Autodesk Inventor part; units mm, degrees
ref_plane "YZ Plane" through (0, 0, 0) normal (1, 0, 0) x (0, 1, 0)
ref_plane "XZ Plane" through (0, 0, 0) normal (0, 1, 0) x (-1, 0, 0)
ref_plane "XY Plane" through (0, 0, 0) normal (0, 0, 1) x (1, 0, 0)
sketch "Szkic2" plane through (0, 0, 0) normal (0, 1, 0) x (-1, 0, 0)
  circle A0 centre (0, 0) radius 11
  circle A1 centre (0, 0) radius 16
  dimension "d0" = 22
  dimension "d1" = 5
extrude "Wyciągnięcie proste1" add sketch "Szkic2" along normal blind 10
sketch "Szkic4" plane through (0, 0, 0) normal (0, 0, 1) x (1, 0, 0)
  line L0 (0, 0) -> (-30, 0)
  line L1 (-30, 0) -> (-30, 10)
  line L2 (-30, 10) -> (0, 10)
  line L3 (0, 10) -> (0, 0)
  line L4 (-30, 0) -> (-40, 0)
  line L5 (-40, 0) -> (-40, 84.8)
  line L6 (-40, 84.8) -> (-30, 84.8)
  line L7 (-30, 84.8) -> (-30, 0)
  dimension "d7" = 84.8
  dimension "d8" = 30
  dimension "d9" = 10
  dimension "d10" = 10
extrude "Wyciągnięcie proste2" add sketch "Szkic4" along normal mid plane 10
fillet "Zaokrąglenie1" radius 20 2 edges at (-40, 0, 0) (-30, 10, 0)
sketch "Szkic7" plane through (-30, 84.8, 5) normal (1, 0, 0) x (0, 0, -1)
  line L0 (10, 0) -> (0, 0)
  circle A0 centre (5, 0) radius 11
  circle A1 centre (5, 0) radius 16
  point P0 (5, -84.8)
  dimension "d14" = 22
  dimension "d15" = 32
extrude "Wyciągnięcie proste3" add sketch "Szkic7" against normal blind 10
sketch "Szkic8" plane through (0, 10, 0) normal (0, 1, 0) x (1, 0, 0)
  circle A0 centre (0, 0) radius 11
extrude "Wyciągnięcie proste4" cut sketch "Szkic8" against normal blind 10
sketch "Szkic9" plane through (0, 10, 0) normal (0, -1, 0) x (1, 0, 0)
  circle A0 centre (0, 0) radius 11
extrude "Wyciągnięcie proste5" cut sketch "Szkic9" against normal blind 10
sketch "Szkic10" plane through (-30, 30, 5) normal (1, 0, 0) x (0, 0, -1)
  line L0 (10, 54.8) -> (0, 54.8)
  circle A0 centre (5, 54.8) radius 11
  point P0 (5, -30)
extrude "Wyciągnięcie proste6" cut sketch "Szkic10" against normal blind 10
properties part number "Gora-gora-ramie"
Work out the finished part from the listing and answer in its coordinate system (mm). A direction names the side the tool comes from. Coordinates: 2 decimals unless noted, no trailing zeros. Write each loop counter-clockwise with the first axis right and the second up, starting at its lowest first coordinate (ties: lowest second). Pieces come first, ordered by that corner, then holes. Notation, with made-up numbers: M 72,80.5 L 126,80.5 A23 ccw 126,98.5 Z; hole C -6.5,-8 d9. An arc over 180 degrees is marked long. Write item = value, one per line.
1. Flat-ended cylindrical pins translate along their axes: pin 1 (5 mm diameter, centred on y = 10.5, z = 10.5, fed in from +X); pin 2 (8 mm diameter, centred on x = 8, z = 1.5, fed in from +Y); pin 3 (17.5 mm diameter, centred on x = 0, z = 0, fed in from +Y); pin 4 (20 mm diameter, centred on x = -28, y = 48, fed in from +Z). Find the tip coordinate at first contact, or state that the pin passes through.
Solution:
pin_1 = 13.83
pin_2 = 10
pin_3 = through
pin_4 = 5
2. The part is cut by section D-D (z = -8). Determine the outline of the cut face in (x, y), then the cut area to 3 significant figures.
Solution:
outline = M -40,70.94 L -30,70.94 L -30,77.25 L -40,77.25 Z; M -40,92.35 L -30,92.35 L -30,98.66 L -40,98.66 Z; M -13.86,0 L -7.55,0 L -7.55,10 L -10,10 A20 cw -13.86,10.38 Z; M 7.55,0 L 13.86,0 L 13.86,10 L 7.55,10 Z
area = 253 mm2
3. Determine the mould class of faces 4 (the face through (-34.93, 100.787, -0.632)), 5 (the face through (-40, 61, 0)), 6 (the face through (-7.1, 4.9, 8.4)) for opening direction Z: released by +Z, released by -Z, zero draft, split by the parting line, or undercut.
Solution:
face_4 = split by the parting line
face_5 = zero draft
face_6 = undercut
4. The part is cut by section B-B (y = 84.8). Determine the outline of the cut face in (x, z).
Solution:
outline = M -40,-16 L -30,-16 L -30,-11 L -40,-11 Z; M -40,11 L -30,11 L -30,16 L -40,16 Z
5. The part is cut by section A-A (z = 0). Determine the outline of the cut face in (x, y).
Solution:
outline = M -40,20 A20 ccw -20,0 L -11,0 L -11,10.03 A20 cw -30,30 L -30,73.8 L -40,73.8 Z; M -40,95.8 L -30,95.8 L -30,100.8 L -40,100.8 Z; M 11,0 L 16,0 L 16,10 L 11,10 Z
6. The part is cut by section C-C (x = 0). Determine the outline of the cut face in (y, z), then the cut area to 3 significant figures.
Solution:
outline = M 0,-16 L 10,-16 L 10,-11 L 0,-11 Z; M 0,11 L 10,11 L 10,16 L 0,16 Z
area = 100 mm2
7. For faces 1 (the face through (-31, 35, -5)), 2 (the face through (-30, 66, 0)), 3 (the face through (-31, 35, 5)), determine the directions among +Z, -Z, +X, -X, +Y, -Y from which every point of the face is accessible in a straight line to the end or side of a thin tool.
Solution:
face_1 = -Z, -X, -Y
face_2 = +Z, -Z, +X, +Y
face_3 = +Z, -X, -Y
8. Straight lines are drawn through the part: line 1 (Z direction, x = 0, y = 6.5); line 2 (X direction, y = 67.5, z = -4.5); line 3 (Y direction, x = 5.5, z = 13). For each, find the intervals that lie inside material, in ascending order. Write a range as from..to.
Solution:
line_1 = -16..-11, 11..16
line_2 = -40..-30
line_3 = 0..10
